```python
from build123d import *
from build123d.topology import SkipClean

# Parameters (mm, degrees)
SKETCH1_R           = 30
SKETCH1_R_2         = 2.1
BOSS_EXTRUDE1_DEPTH = 5
SKETCH7_R           = 4
CUT_EXTRUDE2_DEPTH  = 2
BOSS_EXTRUDE5_DEPTH = 16
SKETCH8_R           = 3.2
CUT_EXTRUDE3_DEPTH  = 65.420493634
CUT_EXTRUDE4_REACH  = 51.295
CUT_EXTRUDE5_REACH  = 61.582
BOSS_EXTRUDE8_DEPTH = 3
CUT_EXTRUDE8_START  = -2
CUT_EXTRUDE8_DEPTH  = 2
SKETCH14_R          = 2
BOSS_EXTRUDE9_DEPTH = 4


with BuildPart() as part:
    # Sketch1 → Boss-Extrude1 (new body)
    with BuildSketch(Plane(origin=(0, 0, 0), x_dir=(1, 0, 0), z_dir=(0, 1, 0))):
        with Locations(Location((0, 0, 0), (0, 0, 270))):
            Circle(SKETCH1_R)
        with Locations(Location((0, 15, 0), (0, 0, 270))):
            Circle(SKETCH1_R_2, mode=Mode.SUBTRACT)
        with Locations(Location((12.990381057, -7.5, 0), (0, 0, 270))):
            Circle(SKETCH1_R_2, mode=Mode.SUBTRACT)
        with Locations(Location((-12.990381057, -7.5, 0), (0, 0, 270))):
            Circle(SKETCH1_R_2, mode=Mode.SUBTRACT)
    extrude(amount=BOSS_EXTRUDE1_DEPTH)

    # Sketch7 → Cut-Extrude2 (cut)
    with BuildSketch(Plane(origin=(0, 5, 0), x_dir=(1, 0, 0), z_dir=(0, 1, 0))):
        with Locations(Location((0, 15, 0), (0, 0, 270))):
            Circle(SKETCH7_R)
        with Locations(Location((12.990381057, -7.5, 0), (0, 0, 270))):
            Circle(SKETCH7_R)
        with Locations(Location((-12.990381057, -7.5, 0), (0, 0, 270))):
            Circle(SKETCH7_R)
    extrude(amount=-CUT_EXTRUDE2_DEPTH, mode=Mode.SUBTRACT)

    # Sketch2 → Boss-Extrude5 (add)
    with BuildSketch(Plane(origin=(0, 5, 0), x_dir=(1, 0, 0), z_dir=(0, 1, 0))):
        with BuildLine():
            Line((23, -19.261360284), (23, 19.261360284))
            ThreePointArc((23, 19.261360284), (20.18526342, 22.193583322), (17, 24.718414189))
            Line((17, 24.718414189), (17, -24.718414189))
            ThreePointArc((17, -24.718414189), (20.18526342, -22.193583322), (23, -19.261360284))
        make_face()
        with BuildLine():
            Line((9, -28.618176043), (9, 28.618176043))
            ThreePointArc((9, 28.618176043), (6.798137481, 29.219605178), (4.556921938, 29.651888008))
            Line((4.556921938, 29.651888008), (4.556921938, 13.6966679))
            Line((4.556921938, 13.6966679), (3, 11))
            Line((3, 11), (3, -29.849623113))
            ThreePointArc((3, -29.849623113), (6.031510215, -29.387427321), (9, -28.618176043))
        make_face()
    boss_extrude5 = extrude(amount=BOSS_EXTRUDE5_DEPTH)

    # Sketch8 → Cut-Extrude3 (cut, through all)
    with BuildSketch(Plane(origin=(23, 0, 0), x_dir=(0, 0, -1), z_dir=(1, 0, 0))):
        with Locations((0, 13.8)):
            Circle(SKETCH8_R)
    cut_extrude3 = extrude(amount=-CUT_EXTRUDE3_DEPTH, mode=Mode.SUBTRACT)

    # Sketch9 → Cut-Extrude4 (cut, up to next)
    with BuildSketch(Plane.ZY.offset(-3), mode=Mode.PRIVATE) as cut_extrude4_sk1:
        Polygon((-29.651888008, 21), (-29.651888008, 5.113260013), (-11, 15.796811053), (-11, 21), (-13.6966679, 21), align=None)
    cut_extrude4_tool1 = extrude(cut_extrude4_sk1.sketch, amount=-CUT_EXTRUDE4_REACH, mode=Mode.PRIVATE) & part.part
    # Sketch9 → Cut-Extrude4 (cut, up to next)
    with BuildSketch(Plane.ZY.offset(-3), mode=Mode.PRIVATE) as cut_extrude4_sk2:
        with BuildLine():
            Line((-11, 21), (-11, 15.796811053))
            Line((-11, 15.796811053), (-3.578594408, 20.047692539))
            ThreePointArc((-3.578594408, 20.047692539), (-1.851568785, 20.757851179), (-5.9e-08, 21))
            Line((-5.9e-08, 21), (-11, 21))
        make_face()
    cut_extrude4_tool2 = extrude(cut_extrude4_sk2.sketch, amount=-CUT_EXTRUDE4_REACH, mode=Mode.PRIVATE) & part.part
    # Sketch9 → Cut-Extrude4 (cut, up to next)
    with BuildSketch(Plane.ZY.offset(-3), mode=Mode.PRIVATE) as cut_extrude4_sk3:
        with BuildLine():
            Line((29.849623113, 21), (-5.9e-08, 21))
            ThreePointArc((-5.9e-08, 21), (1.851568727, 20.757851195), (3.578594408, 20.047692539))
            Line((3.578594408, 20.047692539), (29.849623113, 5))
            Line((29.849623113, 5), (29.849623113, 21))
        make_face()
    cut_extrude4_tool3 = extrude(cut_extrude4_sk3.sketch, amount=-CUT_EXTRUDE4_REACH, mode=Mode.PRIVATE) & part.part
    cut_extrude4_1 = cut_extrude4_tool1.solids().sort_by_distance((3, 15.276519, -21.900696))[0]
    add(cut_extrude4_1, mode=Mode.SUBTRACT)
    cut_extrude4_2 = cut_extrude4_tool2.solids().sort_by_distance((3, 19.285722, -7.892308))[0]
    add(cut_extrude4_2, mode=Mode.SUBTRACT)
    cut_extrude4_3 = cut_extrude4_tool3.solids().sort_by_distance((3, 15.673845, 20.512344))[0]
    add(cut_extrude4_3, mode=Mode.SUBTRACT)
    cut_extrude4 = cut_extrude4_1 + cut_extrude4_2 + cut_extrude4_3  # Cut-Extrude4 as one shape, for the pattern or mirror that repeats it

    # Sketch10 → Cut-Extrude5 (cut, up to next)
    with BuildSketch(Plane.ZY.offset(-17), mode=Mode.PRIVATE) as cut_extrude5_sk1:
        with BuildLine():
            Line((-24.718414189, 21), (-24.718414189, 5))
            Line((-24.718414189, 5), (-4.183421259, 19.659947659))
            ThreePointArc((-4.183421259, 19.659947659), (-2.196403521, 20.656807681), (0, 21))
            Line((0, 21), (-24.718414189, 21))
        make_face()
    cut_extrude5_tool1 = extrude(cut_extrude5_sk1.sketch, amount=-CUT_EXTRUDE5_REACH, mode=Mode.PRIVATE) & part.part
    # Sketch10 → Cut-Extrude5 (cut, up to next)
    with BuildSketch(Plane.ZY.offset(-17), mode=Mode.PRIVATE) as cut_extrude5_sk2:
        with BuildLine():
            Line((4.183421259, 19.659947659), (24.718414189, 5))
            Line((24.718414189, 5), (24.718414189, 21))
            Line((24.718414189, 21), (0, 21))
            ThreePointArc((0, 21), (2.196403521, 20.656807681), (4.183421259, 19.659947659))
        make_face()
    cut_extrude5_tool2 = extrude(cut_extrude5_sk2.sketch, amount=-CUT_EXTRUDE5_REACH, mode=Mode.PRIVATE) & part.part
    cut_extrude5_1 = cut_extrude5_tool1.solids().sort_by_distance((17, 15.681733, -17.202981))[0]
    add(cut_extrude5_1, mode=Mode.SUBTRACT)
    cut_extrude5_2 = cut_extrude5_tool2.solids().sort_by_distance((17, 15.681733, 17.202981))[0]
    add(cut_extrude5_2, mode=Mode.SUBTRACT)
    cut_extrude5 = cut_extrude5_1 + cut_extrude5_2  # Cut-Extrude5 as one shape, for the pattern or mirror that repeats it

    # Mirror1: Boss-Extrude5, Cut-Extrude3, Cut-Extrude4, Cut-Extrude5 across plane
    with SkipClean():  # the faces are left unmerged after this step: merging them gives an invalid solid
        add(boss_extrude5.mirror(Plane.ZY))
        add(cut_extrude3.mirror(Plane.ZY), mode=Mode.SUBTRACT)
        add(cut_extrude4.mirror(Plane.ZY), mode=Mode.SUBTRACT)
        add(cut_extrude5.mirror(Plane.ZY), mode=Mode.SUBTRACT)

    # Sketch13 → Boss-Extrude8 (add)
    with SkipClean():  # the faces are left unmerged after this step: merging them gives an invalid solid
        with BuildSketch(Plane.XZ):
            with BuildLine():
                ThreePointArc((12.385089192, -31.30324211), (15.3125, -31.472644372), (16.98597293, -29.064757431))
                Line((16.98597293, -29.064757431), (17.437516579, -24.411739298))
                ThreePointArc((17.437516579, -24.411739298), (13.125, -26.976552319), (8.445332472, -28.786739298))
                Line((8.445332472, -28.786739298), (12.385089192, -31.30324211))
            make_face()
        boss_extrude8 = extrude(amount=-BOSS_EXTRUDE8_DEPTH)

    # Sketch15 → Cut-Extrude8 (cut)
    with SkipClean():  # the faces are left unmerged after this step: merging them gives an invalid solid
        with BuildSketch(Plane(origin=(0, 5, 0), x_dir=(1, 0, 0), z_dir=(0, 1, 0)).offset(CUT_EXTRUDE8_START)):
            with BuildLine():
                ThreePointArc((15.036417377, 25.959702472), (13.125, 26.976552319), (11.145223248, 27.852899288))
                ThreePointArc((11.145223248, 27.852899288), (12.6875, 26.077333908), (15.036417377, 25.959702472))
            make_face()
            with BuildLine():
                ThreePointArc((17, 28.77498914), (13.533272165, 31.738460943), (11.145223248, 27.852899288))
                ThreePointArc((11.145223248, 27.852899288), (13.125, 26.976552319), (15.036417377, 25.959702472))
                ThreePointArc((15.036417377, 25.959702472), (16.460614977, 27.058779964), (17, 28.77498914))
            make_face()
        cut_extrude8 = extrude(amount=CUT_EXTRUDE8_DEPTH, mode=Mode.SUBTRACT)

    # Sketch14 → Boss-Extrude9 (add)
    with SkipClean():  # the faces are left unmerged after this step: merging them gives an invalid solid
        with BuildSketch(Plane(origin=(0, 3, 0), x_dir=(1, 0, 0), z_dir=(0, 1, 0))):
            with Locations(Location((14, 28.77498914, 0), (0, 0, 90))):
                Circle(SKETCH14_R)
        boss_extrude9 = extrude(amount=BOSS_EXTRUDE9_DEPTH)

    # Mirror2: Boss-Extrude8, Cut-Extrude8, Boss-Extrude9 across plane
    with SkipClean():  # the faces are left unmerged after this step: merging them gives an invalid solid
        add(boss_extrude8.mirror(Plane.ZY))
        add(cut_extrude8.mirror(Plane.ZY), mode=Mode.SUBTRACT)
        add(boss_extrude9.mirror(Plane.ZY))


solid = part.part
```
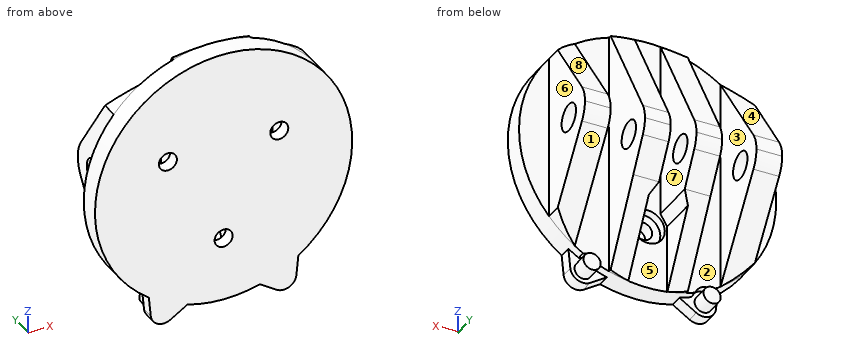
Part model, mm, in its own coordinate system. Face numbers are marked on the shaded views. A direction names the side the tool comes from. Round coordinates to 2 decimals unless told otherwise and drop trailing zeros. Order: outer loops, then holes, each group sorted by start corner. A loop starts at its lowest first (then second) coordinate and runs counter-clockwise, first axis right, second up. Notation, with made-up numbers: M 71,70 L 126,70 A15 cw 126,80 Z; hole C 32,-10.75 d4. An arc over 180 degrees is marked long. Answer in a Markdown table with one row per item. Add a question column.
Q1. Wall check: L1, parallel to X at y = 8.5, z = 13.5; L2, parallel to X at y = 7.25, z = 20; L3, parallel to X at y = 9.5, z = 19. Give the ranges that are in metal, low to high. Write a range as from..to.
Q2. Cut at A-A on x = 0. Give the cut face in (y, z), and give its area (3 significant figures).
Q3. Cut at D-D on z = 21. Give the cut face in (x, y).
Q4. Pin check, flat tips, straight feed: pin 1 (10 mm diameter, centred on x = 20, y = 4.5, fed in from -Z); pin 2 (8 mm diameter, centred on y = 13, z = 9, fed in from +X); pin 3 (4 mm diameter, centred on x = -14.5, z = 9, fed in from +Y). Stop position of each tip, or through.
Q5. Mould opens along X. For the marked faces 5, 6, 7 and 8 say: +X half, -X half, draft (parallel to the pull), parting line (faces both ways), or undercut.
Q6. Cut at C-C on z = -15. Give the cut face in (x, y).
Q7. 3-axis set-ups, long thin cutter, end or side, ignore diameter. For the marked faces 1, 2, 3 and 4: which of +Z, -Z, +X, -X, +Y, -Y reach the whole face in a straight line?
Q8. Cut at B-B on y = 4.25. Give the cut face in (x, z).
Established:
| question | item | result |
|---|---|---|
| 1 | L1 | x = -23..-17, -9..-3, 3..9, 17..23 |
| 1 | L2 | x = -22.36..-17, -9..-3, 3..9, 17..22.36 |
| 1 | L3 | x = -9..-3, 3..9 |
| 2 | outline | M 0,-30 L 5,-30 L 5,-19 L 3,-19 L 3,-17.1 L 0,-17.1 Z; M 0,-12.9 L 3,-12.9 L 3,-11 L 5,-11 L 5,30 L 0,30 Z |
| 2 | area | 271 mm2 |
| 3 | outline | M -21.42,0 L 21.42,0 L 21.42,7.65 L 17,7.65 L 17,5 L 9,5 L 9,10.07 L 3,10.07 L 3,5 L -3,5 L -3,10.07 L -9,10.07 L -9,5 L -17,5 L -17,7.65 L -21.42,7.65 Z |
| 4 | pin 1 | stops at z = -31.51 |
| 4 | pin 2 | stops at x = 23 |
| 4 | pin 3 | stops at y = 5 |
| 5 | face 5 | undercut |
| 5 | face 6 | +X half |
| 5 | face 7 | undercut |
| 5 | face 8 | draft |
| 6 | outline | M -25.98,0 L -2.1,0 L -2.1,3 L -4,3 L -4,5 L -4.56,5 L -4.56,13.51 L -9,13.51 L -9,5 L -17,5 L -17,11.94 L -23,11.94 L -23,5 L -25.98,5 Z; M 2.1,0 L 25.98,0 L 25.98,5 L 23,5 L 23,11.94 L 17,11.94 L 17,5 L 9,5 L 9,13.51 L 4.56,13.51 L 4.56,5 L 4,5 L 4,3 L 2.1,3 Z |
| 7 | face 1 | -Z, +X, +Y |
| 7 | face 2 | +Z, +Y |
| 7 | face 3 | +Z, -Z, +Y |
| 7 | face 4 | +Z, -X, +Y |
| 8 | outline | C -14,-28.77 d4; M -15.04,-25.96 A3 cw -11.15,-27.85 A30 ccw 11.15,-27.85 A3 cw 15.04,-25.96 A30 ccw long Z; C 14,-28.77 d4; hole C -12.99,7.5 d8; hole C 0,-15 d8; hole C 12.99,7.5 d8 |
